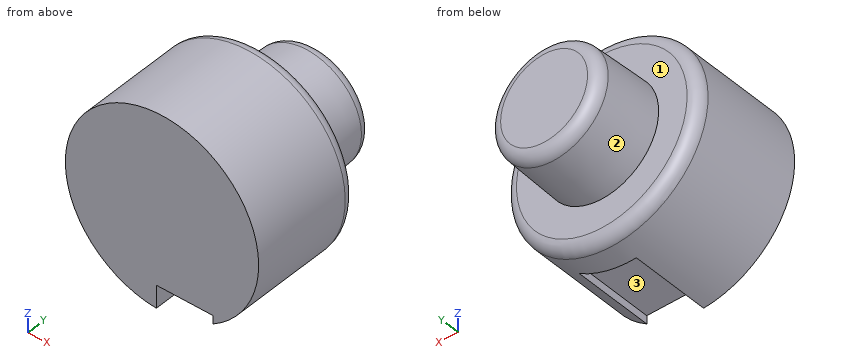
```python
from build123d import *

# Parameters (mm, degrees)
SKETCH1_R           = 8.5
BOSS_EXTRUDE1_DEPTH = 6
FILLET2_R           = 1
SKETCH2_R           = 5
BOSS_EXTRUDE3_DEPTH = 6
BOSS_EXTRUDE3_TAPER = 2
FILLET4_R           = 1
BOSS_EXTRUDE4_START = 4
BOSS_EXTRUDE4_DEPTH = 4
CUT_EXTRUDE4_DEPTH  = 7
SKETCH7_W           = 5.003622488
SKETCH7_H           = 7
BOSS_EXTRUDE5_DEPTH = 8


with BuildPart() as part:
    # Sketch1 → Boss-Extrude1 (new body)
    with BuildSketch(Plane(origin=(0, 0, 0), x_dir=(1, 0, 0), z_dir=(0, 1, 0))):
        with Locations(Location((-51.120170416, 0, 0), (0, 0, 270))):
            Circle(SKETCH1_R)
    extrude(amount=BOSS_EXTRUDE1_DEPTH)

    # Fillet2
    fillet2_edges = [part.edges().sort_by_distance(p)[0] for p in [
        (-51.120170416, 6, -8.5),
    ]]
    fillet(fillet2_edges, radius=FILLET2_R)

    # Sketch2 → Boss-Extrude3 (add)
    with BuildSketch(Plane(origin=(0, 6, 0), x_dir=(1, 0, 0), z_dir=(0, 1, 0))):
        with Locations((-51.120170416, 0)):
            Circle(SKETCH2_R)
    extrude(amount=BOSS_EXTRUDE3_DEPTH, taper=BOSS_EXTRUDE3_TAPER)

    # Fillet4
    fillet4_edges = [part.edges().sort_by_distance(p)[0] for p in [
        (-55.9106458, 12, 0),
    ]]
    fillet(fillet4_edges, radius=FILLET4_R)

    # Sketch3 → Boss-Extrude4 (add)
    with BuildSketch(Plane.XZ.offset(BOSS_EXTRUDE4_START)):
        with BuildLine():
            Line((-51.620170416, 0), (-59.620170416, 0))
            ThreePointArc((-59.620170416, 0), (-57.304828855, -5.830951895), (-51.620170416, -8.485281374))
            Line((-51.620170416, -8.485281374), (-51.620170416, 0))
        make_face()
        with BuildLine():
            ThreePointArc((-42.620170416, 0), (-51.120170416, 8.5), (-59.620170416, 0))
            Line((-59.620170416, 0), (-51.620170416, 0))
            Line((-51.620170416, 0), (-51.620170416, 1.514718626))
            Line((-51.620170416, 1.514718626), (-46.616547928, 1.514718626))
            Line((-46.616547928, 1.514718626), (-46.616547928, 0))
            Line((-46.616547928, 0), (-42.620170416, 0))
        make_face()
        with BuildLine():
            ThreePointArc((-46.616547928, -7.208840717), (-43.686100497, -4.121238215), (-42.620170416, 0))
            Line((-42.620170416, 0), (-46.616547928, 0))
            Line((-46.616547928, 0), (-46.616547928, -7.208840717))
        make_face()
    extrude(amount=-BOSS_EXTRUDE4_DEPTH)

    # Sketch6 → Cut-Extrude4 (cut)
    with BuildSketch(Plane.XZ.offset(4)):
        with BuildLine():
            ThreePointArc((-46.616547928, -7.208840717), (-49.019081783, -8.236226475), (-51.620170416, -8.485281374))
            Line((-51.620170416, -8.485281374), (-51.620170416, 1.514718626))
            Line((-51.620170416, 1.514718626), (-46.616547928, 1.514718626))
            Line((-46.616547928, 1.514718626), (-46.616547928, -7.208840717))
        make_face()
    extrude(amount=-CUT_EXTRUDE4_DEPTH, mode=Mode.SUBTRACT)

    # Sketch7 → Boss-Extrude5 (add)
    with BuildSketch(Plane(origin=(0, 0, 1.514718626), x_dir=(-1, 0, 0), z_dir=(0, 0, -1))):
        with Locations((49.118359172, -0.5)):
            Rectangle(SKETCH7_W, SKETCH7_H)
    extrude(amount=BOSS_EXTRUDE5_DEPTH)


solid = part.part
```
Input: part model. Units: mm. Frame: model coordinates. Face numbers are marked on the shaded views. Give positions to 0.01 mm unless a question says otherwise; leave off trailing zeros. Order: outer loops, then holes, each group sorted by start corner. A loop starts at its lowest first (then second) coordinate and runs counter-clockwise, first axis right, second up.
1. Cut plane B-B (y = 5.5). Return loops of the section in (x, z).
Computed:
outline: circle Ø16.73 at (-51.12, 0)
2. Line query: probe 1 along Z at (x, y) = (-55.5, 4.75); probe 2 along Z at (x, y) = (-52.5, -2.5); probe 3 along X at (y, z) = (1.5, -6.25). Output: solid intervals per line, ascending.
Computed:
probe 1: z = -7.28 to 7.28
probe 2: z = -8.39 to 8.39
probe 3: x = -56.88 to -45.36
3. Pin query (flat end, axial travel): pin 1 Ø0.6 at (y, z) = (1, -7) entering from +X; pin 2 Ø1 at (x, z) = (-48, -7.5) entering from -Y; pin 3 Ø2 at (y, z) = (5.5, 3) entering from -X. Return the tip coordinate at first contact, or that it passes through.
Computed:
pin 1: stops at x = -45.89
pin 2: stops at y = 3
pin 3: stops at x = -59.36
4. Draft query along X for the marked faces 1, 2 and 3. Return one class per face: released by +X, released by -X, zero draft, split by the parting line, or undercut.
Computed:
face 1: zero draft
face 2: split by the parting line
face 3: undercut
5. Cut plane A-A (y = 2). Return loops of the section in (x, z), and give its area (3 significant figures).
Computed:
outline: (-51.62, -8.49) - (-51.62, -6.49) - (-46.62, -6.49) - (-46.62, -7.21) arc R8.5 ccw (long way) to start
area: 219 mm2
